Model file for the job. Use its own axes, mm. A direction names the side the tool comes from. Round coordinates to 2 decimals unless told otherwise and drop trailing zeros. Order: outer loops, then holes, each group sorted by start corner. A loop starts at its lowest first (then second) coordinate and runs counter-clockwise, first axis right, second up. Notation, with made-up numbers: (12, 43) - (31, 43) arc R14 ccw to (31, 49) - close; hole circle Ø1 at (61.5, 66). An arc over 180 degrees is marked (long way). Use one line per item in the form item = value.
from build123d import *

# Parameters (mm, degrees)
F1_DEPTH       = 50.8
F3_D           = 13.49248
F3_CSINK_D     = 23.8252
F3_CSINK_ANGLE = 82
F4_R           = 6.35
F5_SIZE        = 0.8128
F7_D           = 25.4


with BuildPart() as f1:
    # F0 (on Front) → F1 (new body, symmetric)
    with BuildSketch(Plane.XZ):
        Polygon((-6.35, 25.4), (-50.8, 25.4), (-50.8, -25.4), (50.8, -25.4), (50.8, 25.4), (6.35, 25.4), (6.35, 19.05), (-6.35, 19.05), align=None)
    extrude(amount=F1_DEPTH, both=True)

    # F3 (through all)
    with Locations(Plane.XY.offset(25.4)):
        with Locations((-31.75, 31.75), (31.75, 31.75), (31.75, -31.75), (-31.75, -31.75)):
            CounterSinkHole(F3_D / 2, F3_CSINK_D / 2, counter_sink_angle=F3_CSINK_ANGLE)

    # F4
    f4_edges = [f1.edges().sort_by_distance(p)[0] for p in [
        (50.8, -50.8, 0),
        (-50.8, -50.8, 0),
        (-50.8, 50.8, 0),
        (50.8, 50.8, 0),
    ]]
    fillet(f4_edges, radius=F4_R)

    # F5
    f5_edges = [f1.edges().sort_by_distance(p)[0] for p in [
        (25.4, -50.8, 25.4),
        (-50.8, 0, 25.4),
        (0, 50.8, -25.4),
    ]]
    chamfer(f5_edges, length=F5_SIZE)

    # F7 (through all)
    with Locations(Plane.XZ.offset(50.8)):
        with Locations((0, 0)):
            Hole(F7_D / 2)


solid = f1.part
(1) Slice it at B-B on y = 31.75. Give the cut face in (x, z).
Report:
outline = (-50.8, -24.59) - (-49.99, -25.4) - (-38.5, -25.4) - (-38.5, 19.46) - (-43.66, 25.4) - (-49.99, 25.4) - (-50.8, 24.59) - close; (-25, -25.4) - (25, -25.4) - (25, 19.46) - (19.84, 25.4) - (6.35, 25.4) - (6.35, 19.05) - (-6.35, 19.05) - (-6.35, 25.4) - (-19.84, 25.4) - (-25, 19.46) - close; (38.5, -25.4) - (49.99, -25.4) - (50.8, -24.59) - (50.8, 24.59) - (49.99, 25.4) - (43.66, 25.4) - (38.5, 19.46) - close; hole circle Ø25.4 at (0, 0)
(2) Pin check, flat tips, straight feed: pin 1 (15.5 mm diameter, centred on x = 31.75, y = 31.75, fed in from +Z); pin 2 (4 mm diameter, centred on x = 0, y = -13.5, fed in from +Z). Stop position of each tip, or through.
Report:
pin_1 = 20.61
pin_2 = 19.05
(3) Probe probe 1 along Y at (x, z) = (-31.75, 8); probe 2 along X at (y, z) = (-31, -7); probe 3 along X at (y, z) = (34.5, -21.5). List the from-to ranges inside material, lowest first. Write a range as [from, to].
Report:
probe_1 = [-50.8, -38.5], [-25, 25], [38.5, 50.8]
probe_2 = [-50.8, -38.45], [-25.05, -10.6], [10.6, 25.05], [38.45, 50.8]
probe_3 = [-50.8, -37.91], [-25.59, 25.59], [37.91, 50.8]
(4) Slice it at C-C on x = 31.75. Give the cut face in (y, z), then the cut area to 3 significant figures.
Report:
outline = (-50.8, -24.59) - (-49.99, -25.4) - (-38.5, -25.4) - (-38.5, 19.46) - (-43.66, 25.4) - (-49.99, 25.4) - (-50.8, 24.59) - close; (-25, -25.4) - (25, -25.4) - (25, 19.46) - (19.84, 25.4) - (-19.84, 25.4) - (-25, 19.46) - close; (38.5, -25.4) - (49.99, -25.4) - (50.8, -24.59) - (50.8, 24.59) - (49.99, 25.4) - (43.66, 25.4) - (38.5, 19.46) - close
area = 3,730 mm2
(5) Slice it at D-D on x = 0. Give the cut face in (y, z).
Report:
outline = (-50.8, -24.59) - (-49.99, -25.4) - (49.99, -25.4) - (50.8, -24.59) - (50.8, -12.7) - (-50.8, -12.7) - close; (-50.8, 12.7) - (50.8, 12.7) - (50.8, 19.05) - (-50.8, 19.05) - close
(6) Slice it at A-A on z = 0. Give the cut face in (x, y).
Report:
outline = (-50.8, -44.45) arc R6.35 ccw to (-44.45, -50.8) - (-12.7, -50.8) - (-12.7, 50.8) - (-44.45, 50.8) arc R6.35 ccw to (-50.8, 44.45) - close; (12.7, -50.8) - (44.45, -50.8) arc R6.35 ccw to (50.8, -44.45) - (50.8, 44.45) arc R6.35 ccw to (44.45, 50.8) - (12.7, 50.8) - close; hole circle Ø13.49 at (-31.75, -31.75); hole circle Ø13.49 at (-31.75, 31.75); hole circle Ø13.49 at (31.75, -31.75); hole circle Ø13.49 at (31.75, 31.75)
(7) Pull direction Z, two halves, no side cores. Call faces 1 (the face through (-48.413, -48.501, -25.27)), 2 (the face through (50.8, -1, 0)), 3 (the face through (2.75, 0.71, -12.4)), 4 (the face through (-26.197, 27.492, 19.745)): released by +Z, released by -Z, zero draft, split by the parting line, or undercut.
Report:
face_1 = released by -Z
face_2 = zero draft
face_3 = undercut
face_4 = released by +Z
(8) Tool access for faces 5 (the face through (-48.89, -48.99, -0.34)), 6 (the face through (-6.35, -1, 22)): list every direction of +Z, -Z, +X, -X, +Y, -Y with a clear straight run to the whole face (end or side of a thin tool).
Report:
face_5 = +Z, -Z, -X, -Y
face_6 = +Z, +Y, -Y
